```python
from build123d import *
from OCP.BRepFilletAPI import BRepFilletAPI_MakeChamfer

# Parameters (mm, degrees)
SKETCH39_R               = 12.7
BOSS_EXTRUDE16_DEPTH     = 105.41
CUT_EXTRUDE13_DEPTH      = 297.507996976
CUT_EXTRUDE13_DEPTH_BACK = 297.507996976
SKETCH41_R               = 12.7
BOSS_EXTRUDE17_DEPTH     = 5.461
SKETCH42_R               = 53.594
CUT_EXTRUDE14_DEPTH      = 41.91
SKETCH43_R               = 12.7
CUT_EXTRUDE15_DEPTH      = 41.275
CUT_EXTRUDE25_DEPTH      = 14.224
CHAMFER1_SIZE            = 12.7
CHAMFER1_SIZE2           = 2.239352655
CUT_EXTRUDE18_DEPTH      = 63.5
CUT_REVOLVE4_ANGLE       = 45
CUT_EXTRUDE22_REACH      = 286.32
SKETCH53_R               = 12.7
CUT_EXTRUDE23_DEPTH      = 285.32019658
CUT_EXTRUDE24_DEPTH      = 290.353535308


with BuildPart() as part:
    # Sketch39 → Boss-Extrude16 (new body)
    with BuildSketch(Plane(origin=(0, 0, 0), x_dir=(-1, 0, 0), z_dir=(0, 0, -1))):
        with BuildLine():
            Line((-37.30625, 269.9512), (37.30625, 269.9512))
            ThreePointArc((37.30625, 269.9512), (59.865817558, 256.222785651), (58.039, 229.877649733))
            Line((58.039, 229.877649733), (58.039, 107.49735517))
            ThreePointArc((58.039, 107.49735517), (55.67225609, 95.733970947), (48.940336125, 85.8012))
            ThreePointArc((48.940336125, 85.8012), (0, 54.0512), (-48.940336125, 85.8012))
            ThreePointArc((-48.940336125, 85.8012), (-55.67225609, 95.733970947), (-58.039, 107.49735517))
            Line((-58.039, 107.49735517), (-58.039, 229.877649733))
            ThreePointArc((-58.039, 229.877649733), (-59.865817558, 256.222785651), (-37.30625, 269.9512))
        make_face()
        with Locations((-37.30625, 244.5512)):
            Circle(SKETCH39_R, mode=Mode.SUBTRACT)
        with Locations((37.30625, 244.5512)):
            Circle(SKETCH39_R, mode=Mode.SUBTRACT)
    extrude(amount=BOSS_EXTRUDE16_DEPTH)

    # Sketch40 → Cut-Extrude13 (cut, two sides)
    with BuildSketch(Plane(origin=(0, 0, 0), x_dir=(0, 0, -1), z_dir=(1, 0, 0))) as cut_extrude13_sk:
        with BuildLine():
            Line((99.949, 208.9912), (70.469723816, 127.997554342))
            ThreePointArc((70.469723816, 127.997554342), (65.255767984, 108.538806271), (63.5, 88.470286378))
            Line((63.5, 88.470286378), (63.5, 54.0512))
            Line((63.5, 54.0512), (105.41, 54.0512))
            Line((105.41, 54.0512), (105.41, 229.877649733))
            Line((105.41, 229.877649733), (99.949, 229.877649733))
            Line((99.949, 229.877649733), (99.949, 208.9912))
        make_face()
    extrude(amount=CUT_EXTRUDE13_DEPTH, mode=Mode.SUBTRACT)
    extrude(cut_extrude13_sk.sketch, amount=-CUT_EXTRUDE13_DEPTH_BACK, mode=Mode.SUBTRACT)

    # Sketch41 → Boss-Extrude17 (add)
    with BuildSketch(Plane(origin=(0, 0, -105.41), x_dir=(-1, 0, 0), z_dir=(0, 0, -1))):
        with BuildLine():
            Line((-37.30625, 269.9512), (37.30625, 269.9512))
            ThreePointArc((37.30625, 269.9512), (62.70625, 244.5512), (37.30625, 219.1512))
            Line((37.30625, 219.1512), (-37.30625, 219.1512))
            ThreePointArc((-37.30625, 219.1512), (-62.70625, 244.5512), (-37.30625, 269.9512))
        make_face()
        with Locations((-37.30625, 244.5512)):
            Circle(SKETCH41_R, mode=Mode.SUBTRACT)
        with Locations((37.30625, 244.5512)):
            Circle(SKETCH41_R, mode=Mode.SUBTRACT)
    extrude(amount=-BOSS_EXTRUDE17_DEPTH)

    # Sketch42 → Cut-Extrude14 (cut)
    with BuildSketch(Plane(origin=(0, 0, -105.41), x_dir=(-1, 0, 0), z_dir=(0, 0, -1))):
        with Locations((0, 107.6452)):
            Circle(SKETCH42_R)
    extrude(amount=-CUT_EXTRUDE14_DEPTH, mode=Mode.SUBTRACT)

    # Sketch43 → Cut-Extrude15 (cut)
    with BuildSketch(Plane(origin=(0, 0, -63.5), x_dir=(-1, 0, 0), z_dir=(0, 0, -1))):
        with Locations((0, 107.6452)):
            Circle(SKETCH43_R)
        with BuildLine():
            Line((-17.140551152, 142.338453637), (-8.320140689, 124.485542452))
            ThreePointArc((-8.320140689, 124.485542452), (-8.084797468, 122.315875536), (-9.305565087, 120.50685166))
            ThreePointArc((-9.305565087, 120.50685166), (-15.875, 107.6452), (-9.305565087, 94.78354834))
            ThreePointArc((-9.305565087, 94.78354834), (-8.084797468, 92.974524464), (-8.320140689, 90.804857548))
            Line((-8.320140689, 90.804857548), (-17.140551152, 72.951946363))
            ThreePointArc((-17.140551152, 72.951946363), (-24.663775135, 67.208970871), (-33.791061651, 69.713628025))
            ThreePointArc((-33.791061651, 69.713628025), (-50.8, 107.6452), (-33.791061651, 145.576771975))
            ThreePointArc((-33.791061651, 145.576771975), (-24.663775135, 148.081429129), (-17.140551152, 142.338453637))
        make_face()
    extrude(amount=-CUT_EXTRUDE15_DEPTH, mode=Mode.SUBTRACT)

    # Sketch57 → Cut-Extrude25 (cut)
    with BuildSketch(Plane.XY):
        with BuildLine():
            Line((-58.039, 121.8184), (-51.685948165, 121.8184))
            ThreePointArc((-51.685948165, 121.8184), (0, 161.2392), (51.685948165, 121.8184))
            Line((51.685948165, 121.8184), (58.039, 121.8184))
            Line((58.039, 121.8184), (58.039, 229.877649733))
            ThreePointArc((58.039, 229.877649733), (59.865817558, 256.222785651), (37.30625, 269.9512))
            Line((37.30625, 269.9512), (-37.30625, 269.9512))
            ThreePointArc((-37.30625, 269.9512), (-59.865817558, 256.222785651), (-58.039, 229.877649733))
            Line((-58.039, 229.877649733), (-58.039, 121.8184))
        make_face()
    extrude(amount=-CUT_EXTRUDE25_DEPTH, mode=Mode.SUBTRACT)

    # Chamfer1: one chamfer whose edges measure the first distance from different faces: ONE call of the kernel's chamfer builder (chamfer() names one face for all edges)
    chamfer1_edges_1 = [part.edges().sort_by_distance(p)[0] for p in [
        (58.039, 175.848024867, -14.224),
    ]]
    chamfer1_side_1 = [part.faces().sort_by_distance(p)[0] for p in [
        (58.039, 173.156318685, -49.465514594),
    ]]
    chamfer1_edges_2 = [part.edges().sort_by_distance(p)[0] for p in [
        (-58.039, 175.848024867, -14.224),
    ]]
    chamfer1_side_2 = [part.faces().sort_by_distance(p)[0] for p in [
        (-58.039, 173.156318685, -49.465514594),
    ]]
    chamfer1_edges_3 = [part.edges().sort_by_distance(p)[0] for p in [
        (-59.865817558, 256.222785651, -14.224),
    ]]
    chamfer1_side_3 = [part.faces().sort_by_distance(p)[0] for p in [
        (-59.865817558, 256.222785651, -57.0865),
    ]]
    chamfer1_edges_4 = [part.edges().sort_by_distance(p)[0] for p in [
        (0, 269.9512, -14.224),
    ]]
    chamfer1_side_4 = [part.faces().sort_by_distance(p)[0] for p in [
        (0, 269.9512, -57.0865),
    ]]
    chamfer1_edges_5 = [part.edges().sort_by_distance(p)[0] for p in [
        (59.865817558, 256.222785651, -14.224),
    ]]
    chamfer1_side_5 = [part.faces().sort_by_distance(p)[0] for p in [
        (59.865817558, 256.222785651, -57.0865),
    ]]
    chamfer1 = BRepFilletAPI_MakeChamfer(part.part.solid().wrapped)
    for e in chamfer1_edges_1:
        chamfer1.Add(CHAMFER1_SIZE, CHAMFER1_SIZE2, e.wrapped, chamfer1_side_1[0].wrapped)  # the first distance lies on this face
    for e in chamfer1_edges_2:
        chamfer1.Add(CHAMFER1_SIZE, CHAMFER1_SIZE2, e.wrapped, chamfer1_side_2[0].wrapped)  # the first distance lies on this face
    for e in chamfer1_edges_3:
        chamfer1.Add(CHAMFER1_SIZE, CHAMFER1_SIZE2, e.wrapped, chamfer1_side_3[0].wrapped)  # the first distance lies on this face
    for e in chamfer1_edges_4:
        chamfer1.Add(CHAMFER1_SIZE, CHAMFER1_SIZE2, e.wrapped, chamfer1_side_4[0].wrapped)  # the first distance lies on this face
    for e in chamfer1_edges_5:
        chamfer1.Add(CHAMFER1_SIZE, CHAMFER1_SIZE2, e.wrapped, chamfer1_side_5[0].wrapped)  # the first distance lies on this face
    add(Compound.cast(chamfer1.Shape()), mode=Mode.REPLACE)

    # Sketch46 → Cut-Extrude18 (cut)
    with BuildSketch(Plane(origin=(0, 0, -105.41), x_dir=(-1, 0, 0), z_dir=(0, 0, -1))):
        with BuildLine():
            Line((-56.154391463, 206.4512), (-56.154391463, 123.5202))
            Line((-56.154391463, 123.5202), (-51.188877806, 123.5202))
            ThreePointArc((-51.188877806, 123.5202), (-38.080986117, 145.35667481), (-16.37335621, 158.676857257))
            ThreePointArc((-16.37335621, 158.676857257), (-16.447164367, 159.694072309), (-16.088636924, 160.64886662))
            Line((-16.088636924, 160.64886662), (-32.030251423, 219.1512))
            Line((-32.030251423, 219.1512), (-49.871677642, 219.1512))
            Line((-49.871677642, 219.1512), (-56.154391463, 206.4512))
        make_face()
        with BuildLine():
            Line((56.154391463, 206.4512), (56.154391463, 123.5202))
            Line((56.154391463, 123.5202), (51.188877806, 123.5202))
            ThreePointArc((51.188877806, 123.5202), (38.083220696, 145.354418203), (16.379403996, 158.674916448))
            ThreePointArc((16.379403996, 158.674916448), (16.453052349, 159.697717152), (16.090874379, 160.657077605))
            Line((16.090874379, 160.657077605), (32.030251423, 219.1512))
            Line((32.030251423, 219.1512), (49.871677642, 219.1512))
            Line((49.871677642, 219.1512), (56.154391463, 206.4512))
        make_face()
        with BuildLine():
            Line((28.739484198, 219.1512), (13.027568982, 161.491814117))
            ThreePointArc((13.027568982, 161.491814117), (12.22875634, 160.848818221), (11.773335802, 159.930048667))
            ThreePointArc((11.773335802, 159.930048667), (-0.003175786, 161.239199906), (-11.77953214, 159.928653009))
            ThreePointArc((-11.77953214, 159.928653009), (-12.231981249, 160.842690157), (-13.025331527, 161.483603132))
            Line((-13.025331527, 161.483603132), (-28.739484198, 219.1512))
            Line((-28.739484198, 219.1512), (28.739484198, 219.1512))
        make_face()
    extrude(amount=-CUT_EXTRUDE18_DEPTH, mode=Mode.SUBTRACT)

    # Sketch47 → Cut-Revolve4 (revolve, symmetric, cut)
    with BuildSketch(Plane(origin=(0, 0, 0), x_dir=(0, 0, -1), z_dir=(1, 0, 0))) as cut_revolve4_sk:
        Polygon((99.949, 219.1512), (63.5, 161.085477364), (105.41, 161.085477364), (105.41, 219.1512), align=None)
    revolve(axis=Axis((0, 107.110477364, -63.5), (0, 0, -1)), revolution_arc=CUT_REVOLVE4_ANGLE / 2, mode=Mode.SUBTRACT)
    revolve(cut_revolve4_sk.sketch, axis=Axis((0, 107.110477364, -63.5), (0, 0, 1)), revolution_arc=CUT_REVOLVE4_ANGLE / 2, mode=Mode.SUBTRACT)

    # Sketch52 → Cut-Extrude22 (cut, up to next)
    with BuildSketch(Plane(origin=(0, 0, -63.5), x_dir=(-1, 0, 0), z_dir=(0, 0, -1)), mode=Mode.PRIVATE) as cut_extrude22_sk1:
        with BuildLine():
            Line((-56.154391463, 123.5202), (-51.188877806, 123.5202))
            ThreePointArc((-51.188877806, 123.5202), (-53.59155752, 107.133537422), (-50.876442713, 90.795736718))
            ThreePointArc((-50.876442713, 90.795736718), (-54.826433246, 106.946521771), (-56.154391463, 123.5202))
        make_face()
    cut_extrude22_tool1 = extrude(cut_extrude22_sk1.sketch, amount=CUT_EXTRUDE22_REACH, mode=Mode.PRIVATE) & part.part
    # Sketch52 → Cut-Extrude22 (cut, up to next)
    with BuildSketch(Plane(origin=(0, 0, -63.5), x_dir=(-1, 0, 0), z_dir=(0, 0, -1)), mode=Mode.PRIVATE) as cut_extrude22_sk2:
        with BuildLine():
            Line((51.188877806, 123.5202), (56.154391463, 123.5202))
            ThreePointArc((56.154391463, 123.5202), (54.826433246, 106.946521771), (50.876442713, 90.795736718))
            ThreePointArc((50.876442713, 90.795736718), (53.59155752, 107.133537422), (51.188877806, 123.5202))
        make_face()
    cut_extrude22_tool2 = extrude(cut_extrude22_sk2.sketch, amount=CUT_EXTRUDE22_REACH, mode=Mode.PRIVATE) & part.part
    add(cut_extrude22_tool1.solids().sort_by_distance((54.141808, 115.249163, -63.5))[0], mode=Mode.SUBTRACT)
    add(cut_extrude22_tool2.solids().sort_by_distance((-54.141808, 115.249163, -63.5))[0], mode=Mode.SUBTRACT)

    # Sketch53 → Cut-Extrude23 (cut, through all)
    with BuildSketch(Plane(origin=(0, 0, -63.5), x_dir=(-1, 0, 0), z_dir=(0, 0, -1))):
        with Locations((0, 107.6452)):
            Circle(SKETCH53_R)
    extrude(amount=-CUT_EXTRUDE23_DEPTH, mode=Mode.SUBTRACT)

    # Sketch54 → Cut-Extrude24 (cut, through all)
    with BuildSketch(Plane(origin=(0, 0, -22.225), x_dir=(-1, 0, 0), z_dir=(0, 0, -1))):
        with BuildLine():
            ThreePointArc((-31.581997064, 143.09702472), (-47.47898919, 107.6452), (-31.581997064, 72.19337528))
            ThreePointArc((-31.581997064, 72.19337528), (-21.218076505, 72.791679022), (-21.816380247, 83.155599581))
            ThreePointArc((-21.816380247, 83.155599581), (-32.79778919, 107.6452), (-21.816380247, 132.134800419))
            ThreePointArc((-21.816380247, 132.134800419), (-21.218076505, 142.498720978), (-31.581997064, 143.09702472))
        make_face()
    extrude(amount=-CUT_EXTRUDE24_DEPTH, mode=Mode.SUBTRACT)


solid = part.part
```
Geometry check sheet. Reference: the model listing, model coordinates, mm. A direction names the side the tool comes from. Coordinates: 2 decimals unless noted, no trailing zeros. Order: outer loops, then holes, each group sorted by start corner. A loop starts at its lowest first (then second) coordinate and runs counter-clockwise, first axis right, second up. Notation, with made-up numbers: M 26,71.25 L 81,71.25 A20 ccw 81,105.25 Z; hole C 27,46 d10. An arc over 180 degrees is marked long. One line per question, with ' | ' between items. Start each with the question number.
Item 1: Draft check along Y on faces 5 (the flat face through (-57.188, 169.061, -85.416)), 6 (the cylindrical face through (50.796, 107.046, -43.151)), 7 (the flat face through (-30, 217, -99.949)). Enter one of: pulls with the +Y half, pulls with the -Y half, needs draft (parallel to the pull), parting line crosses it, or undercut.
Item 2: Cross-section at A-A on x = 0. Enter the section's corners in (y, z), then the cut area to 3 significant figures.
Item 3: Material ranges on L1, parallel to Y at x = 0, z = -42.5; L2, parallel to X at y = 119, z = -41; L3, parallel to X at y = 193.5, z = -77, recorded low to high. Write a range as [from, to].
Item 4: Cross-section at C-C on x = 41. State how many separate pieces and enclosed holes the cut face has, then the cut area to 3 significant figures.
Item 5: Set-up check for faces 1 (the cylindrical face through (55.737, 114.208, -65.201)), 2 (the cylindrical face through (21.112, 142.377, -11.268)), 3 (the flat face through (58.039, 168, -49)), 4 (the flat face through (-56.904, 176.975, -20.485)): record each of +Z, -Z, +X, -X, +Y, -Y from which the full face is reachable in a straight line by a thin tool's end or side.
Item 6: Gauge pin test, flat ends, axial feed: pin 1 (8 mm diameter, centred on x = 0, y = 228.5, fed in from +Z); pin 2 (12 mm diameter, centred on y = 84, z = -34.5, fed in from -X); pin 3 (2 mm diameter, centred on x = -23.5, y = 83, fed in from -Z); pin 4 (5 mm diameter, centred on x = 4.5, y = 101, fed in from +Z). Record the tip position at first contact, or that the pin passes through.
Item 7: Cross-section at B-B on z = -86.5. Enter the section's corners in (x, y), then the cut area to 3 significant figures.
Findings:
1) face 5: pulls with the -Y half | face 6: undercut | face 7: needs draft
2) outline: M 54.05,-63.5 L 94.95,-63.5 L 94.95,0 L 54.05,0 Z; M 120.35,-63.5 L 161.24,-63.5 L 161.24,-41.91 L 219.15,-41.91 L 219.15,-105.41 L 269.95,-105.41 L 269.95,-26.92 L 267.71,-14.22 L 161.24,-14.22 L 161.24,0 L 120.35,0 Z | area: 11,400 mm²
3) L1: y = [54.05, 94.95], [120.35, 161.24], [219.15, 269.95] | L2: x = [-58.04, -5.69], [5.69, 11.09], [49.51, 58.04] | L3: x = [-58.04, -56.15], [-25.04, -21.75], [21.75, 25.04], [56.15, 58.04]
4) separate pieces: 3 | enclosed holes: 0 | area: 5,350 mm²
5) face 1: -Z | face 2: +Z, -Z | face 3: +Z, -Z, +X, -Y | face 4: +Z, -X
6) pin 1: stops at z = -14.22 | pin 2: stops at x = -52.5 | pin 3: stops at z = -63.5 | pin 4: passes through
7) outline: M -58.04,172.04 L -56.15,172.04 L -56.15,206.45 L -49.87,219.15 L -32.03,219.15 L -25.22,194.15 A90.62 cw -22.15,194.98 L -28.74,219.15 L 28.74,219.15 L 22.15,194.98 A90.62 cw 25.22,194.15 L 32.03,219.15 L 49.87,219.15 L 56.15,206.45 L 56.15,172.04 L 58.04,172.04 L 58.04,229.88 A25.4 ccw 37.31,269.95 L -37.31,269.95 A25.4 ccw -58.04,229.88 Z; hole C -37.31,244.55 d25.4; hole C 37.31,244.55 d25.4 | area: 5,360 mm²
